Geometry check sheet. Reference: the model listing, model coordinates, mm. Face numbers are marked on the shaded views. A direction names the side the tool comes from. Give positions to 0.01 mm unless a question says otherwise; leave off trailing zeros. Order: outer loops, then holes, each group sorted by start corner. A loop starts at its lowest first (then second) coordinate and runs counter-clockwise, first axis right, second up.
from build123d import *

# Parameters (mm, degrees)
SKETCH1_W           = 30
SKETCH1_H           = 30
SKETCH1_W_2         = 7
SKETCH1_H_2         = 26
BOSS_EXTRUDE3_DEPTH = 90
SKETCH6_R           = 12.35
CUT_EXTRUDE5_DEPTH  = 23
SKETCH8_R           = 3.6
CUT_EXTRUDE6_DEPTH  = 17


with BuildPart() as part:
    # Sketch1 → Boss-Extrude3 (new body)
    with BuildSketch(Plane(origin=(0, 0, 0), x_dir=(0, 0, -1), z_dir=(1, 0, 0))):
        Rectangle(SKETCH1_W, SKETCH1_H)
        with Locations((-9.5, 0)):
            Rectangle(SKETCH1_W_2, SKETCH1_H_2, mode=Mode.SUBTRACT)
        with Locations((9.5, 0)):
            Rectangle(SKETCH1_W_2, SKETCH1_H_2, mode=Mode.SUBTRACT)
    extrude(amount=BOSS_EXTRUDE3_DEPTH)

    # Sketch6 → Cut-Extrude5 (cut)
    with BuildSketch(Plane(origin=(0, 0, -15), x_dir=(-1, 0, 0), z_dir=(0, 0, -1))):
        with Locations((-75, 0)):
            Circle(SKETCH6_R)
    extrude(amount=-CUT_EXTRUDE5_DEPTH, mode=Mode.SUBTRACT)

    # Sketch8 → Cut-Extrude6 (cut)
    with BuildSketch(Plane.XY.offset(15)):
        with Locations((75, 0)):
            Circle(SKETCH8_R)
    extrude(amount=-CUT_EXTRUDE6_DEPTH, mode=Mode.SUBTRACT)


solid = part.part
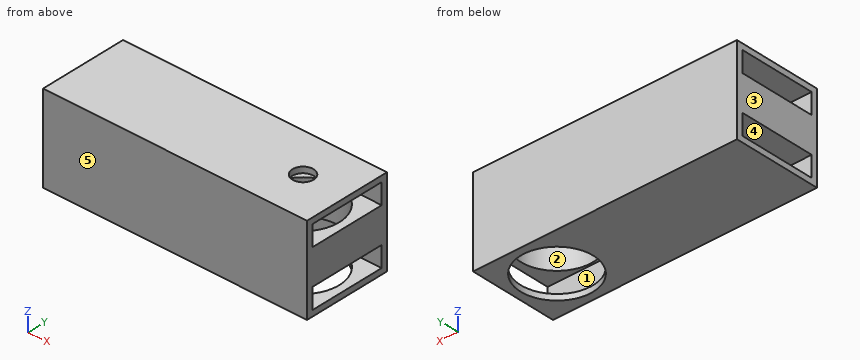
Item 1: Sectioned sample at D-D (x = 43). Enter the section's corners in (y, z).
Reported:
outline: (-15, -15) - (15, -15) - (15, 15) - (-15, 15) - close; hole (-13, -13) - (13, -13) - (13, -6) - (-13, -6) - close; hole (-13, 6) - (13, 6) - (13, 13) - (-13, 13) - close
Item 2: Set-up check for the marked faces 4 and 5: record each of +Z, -Z, +X, -X, +Y, -Y from which the full face is reachable in a straight line by a thin tool's end or side.
Reported:
face 4: +X, -X
face 5: +Z, -Z, +X, -X, -Y
Item 3: Sectioned sample at C-C (x = 75). Enter the section's corners in (y, z).
Reported:
outline: (-15, -15) - (-12.35, -15) - (-12.35, -13) - (-13, -13) - (-13, -6) - (-12.35, -6) - (-12.35, 6) - (-13, 6) - (-13, 13) - (-3.6, 13) - (-3.6, 15) - (-15, 15) - close; (3.6, 13) - (13, 13) - (13, 6) - (12.35, 6) - (12.35, -6) - (13, -6) - (13, -13) - (12.35, -13) - (12.35, -15) - (15, -15) - (15, 15) - (3.6, 15) - close
Item 4: Draft check along X on the marked faces 1, 2 and 3. Enter one of: released by +X, released by -X, zero draft, split by the parting line, or undercut.
Reported:
face 1: zero draft
face 2: undercut
face 3: released by -X
Item 5: Gauge pin test, flat end, axial feed: pin 1 (5 mm diameter, centred on y = 2, z = 1, fed in from -X). Record the tip position at first contact, or that the pin passes through.
Reported:
pin 1: stops at x = 0
Item 6: Sectioned sample at B-B (z = -12). Enter the section's corners in (x, y), and give its area (3 significant figures).
Reported:
outline: (0, -15) - (90, -15) - (90, -13) - (0, -13) - close; (0, 13) - (90, 13) - (90, 15) - (0, 15) - close
area: 360 mm2
Item 7: Scan lines: L1, parallel to Z at x = 53.5, y = -10.75; L2, parallel to Y at x = 8.5, z = -9.75; L3, parallel to Y at x = 75, z = 0.75. Record each from-to range of solid material in increasing order.
Reported:
L1: z = -15 to -13, -6 to 6, 13 to 15
L2: y = -15 to -13, 13 to 15
L3: y = -15 to -12.35, 12.35 to 15
Item 8: Sectioned sample at A-A (y = 0). Enter the section's corners in (x, z).
Reported:
outline: (0, -15) - (62.65, -15) - (62.65, -13) - (0, -13) - close; (0, -6) - (62.65, -6) - (62.65, 6) - (0, 6) - close; (0, 13) - (71.4, 13) - (71.4, 15) - (0, 15) - close; (78.6, 13) - (90, 13) - (90, 15) - (78.6, 15) - close; (87.35, -15) - (90, -15) - (90, -13) - (87.35, -13) - close; (87.35, -6) - (90, -6) - (90, 6) - (87.35, 6) - close
